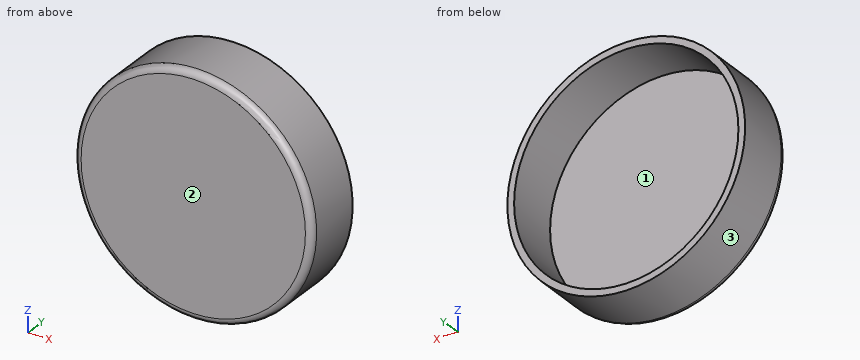
```python
from build123d import *

# Parameters (mm, degrees)
SKETCH1_R           = 53
SKETCH1_R_2         = 50
BOSS_EXTRUDE1_DEPTH = 27
SKETCH1_2_R         = 53
BOSS_EXTRUDE2_DEPTH = 3
FILLET1_R           = 3


with BuildPart() as part:
    # Sketch1 → Boss-Extrude1 (new body)
    with BuildSketch(Plane(origin=(0, 0, 0), x_dir=(1, 0, 0), z_dir=(0, 1, 0))):
        with Locations(Location((0, 0, 0), (0, 0, 270))):
            Circle(SKETCH1_R)
        with Locations(Location((0, 0, 0), (0, 0, 270))):
            Circle(SKETCH1_R_2, mode=Mode.SUBTRACT)
    extrude(amount=BOSS_EXTRUDE1_DEPTH)

    # Sketch1_2 → Boss-Extrude2 (add)
    with BuildSketch(Plane(origin=(0, 0, 0), x_dir=(1, 0, 0), z_dir=(0, 1, 0))):
        with Locations(Location((0, 0, 0), (0, 0, 270))):
            Circle(SKETCH1_2_R)
    extrude(amount=BOSS_EXTRUDE2_DEPTH)

    # Fillet1
    fillet1_edges = [part.edges().sort_by_distance(p)[0] for p in [
        (0, 0, -53),
    ]]
    fillet(fillet1_edges, radius=FILLET1_R)


solid = part.part
```
Build history of the part. All positions in model axes, mm. Face numbers are marked on the shaded views. Round coordinates to 2 decimals unless told otherwise and drop trailing zeros. Loops run counter-clockwise (first coordinate to the right, second up) from the corner with the lowest first, then second, coordinate; pieces in that order, holes last.
Item 1: Saw through at B-B (z = 0). List the corners of the cut face in (x, y).
Item 2: Saw through at A-A (x = 0). List the corners of the cut face in (y, z).
Item 3: Saw through at C-C (y = 22.5). List the corners of the cut face in (x, z).
Item 4: Pin check, flat tips, straight feed: P1, Ø5, axis at x = 21.5, y = 7, coming from the -Z side; P2, Ø12, axis at y = 11.5, z = 34.5, coming from the +X side (3 decimals); P3, Ø2, axis at x = -16, z = 7.5, coming from the +Y side. Stop position of each tip, or through.
Item 5: Drill centre lines: line 1 along X through (y, z) = (15.75, 0); line 2 along Y through (x, z) = (23.5, -9); line 3 along Z through (x, y) = (-19, 16). Where is each one in solid material? Low to high.
Item 6: Two-plate mould, pull along X, no slides. Class the marked faces 1, 2 and 3: released by +X, released by -X, zero draft, split by the parting line, or undercut.
Worked answers:
1. outline: (-53, 3) arc R3 ccw to (-50, 0) - (50, 0) arc R3 ccw to (53, 3) - (53, 27) - (50, 27) - (50, 3) - (-50, 3) - (-50, 27) - (-53, 27) - close
2. outline: (0, -50) arc R3 ccw to (3, -53) - (27, -53) - (27, -50) - (3, -50) - (3, 50) - (27, 50) - (27, 53) - (3, 53) arc R3 ccw to (0, 50) - close
3. outline: circle Ø106 at (0, 0); hole circle Ø100 at (0, 0)
4. P1: stops at z = -49.48
4. P2: stops at x = 44.685
4. P3: stops at y = 3
5. line 1: x = -53 to -50, 50 to 53
5. line 2: y = 0 to 3
5. line 3: z = -49.48 to -46.25, 46.25 to 49.48
6. face 1: undercut
6. face 2: zero draft
6. face 3: split by the parting line
